Solid Edge part; units mm, degrees
sketch "Sketch1" plane through (0, 0, 0) normal (0, 0, 1) x (1, 0, 0)
  circle A0 centre (0, 0) radius 12.7
extrude "Protrusion1" add sketch "Sketch1" along normal blind 38.1
chamfer "Chamfer1" distance 1.905 angle 45 2 edges at (-12.7, 0, 0) (-12.7, 0, 38.1)
sketch "Sketch2" plane through (0, 0, 38.1) normal (0, 0, 1) x (1, 0, 0)
  line L0 (-4.1244, 7.1438) -> (4.1244, 7.1438)
  line L1 (8.2489, 0) -> (4.1244, 7.1437)
  line L2 (4.1244, -7.1437) -> (8.2489, 0)
  line L3 (-4.1244, -7.1438) -> (4.1244, -7.1438)
  line L4 (-8.2489, 0) -> (-4.1244, -7.1437)
  line L5 (-4.1244, 7.1437) -> (-8.2489, 0)
extrude "Cutout1" cut sketch "Sketch2" against normal blind 19.05
properties part number "24104263"
CAD build for the part. Positions are in the model's coordinates, mm. A direction names the side the tool comes from. Round coordinates to 2 decimals unless told otherwise and drop trailing zeros. Loops run counter-clockwise (first coordinate to the right, second up) from the corner with the lowest first, then second, coordinate; pieces in that order, holes last. Notation, with made-up numbers: M 20.25,-27 L 52.25,-27 A6 cw 52.25,-16 Z; hole C -4,63.5 d7. An arc over 180 degrees is marked long. Return JSON: item names as keys, results as strings. Group by question number.
(1) Drop flat-ended pins along their axis: P1, Ø4.5, axis at x = -4, y = -1.5, coming from the +Z side; P2, Ø1, axis at x = -8, z = 19, coming from the +Y side; P3, Ø1.5, axis at y = 7, z = 32, coming from the -X side. Give the stop position or say it passes through.
(2) Saw through at B-B, the plane x = 0. List the corners of the cut face in (y, z) (3 decimals), and give its area (3 significant figures).
(3) Tool access for faces 1 (the flat face through (0, 0, 19.05)), 2 (the conical face through (10.41, 3.28, 0.12)): list every direction of +Z, -Z, +X, -X, +Y, -Y with a clear straight run to the whole face (end or side of a thin tool).
(4) Mould opens along X. For faces 3 (the flat face through (-6.216, -3.522, 28.708)), 4 (the flat face through (7, 3, 38.1)), 5 (the cylindrical face through (-2.75, 12.4, 18.81)) say: +X half, -X half, draft (parallel to the pull), parting line (faces both ways), or undercut.
(5) Wall check: probe 1 along Z at (x, y) = (-3, -5.25); probe 2 along X at (y, z) = (-10.5, 15.5); probe 3 along X at (y, z) = (-3, 29). Give the ranges that are in metal, low to high. Write a range as [from, to].
(6) Saw through at C-C, the plane z = 13. List the corners of the cut face in (x, y).
(7) Saw through at A-A, the plane z = 23. List the corners of the cut face in (x, y), and give its area (3 significant figures).
Answer list:
{
 "1": {"P1": "z = 19.05", "P2": "y = 10.25", "P3": "x = -11.06"},
 "2": {"outline": "M -12.7,1.905 L -10.795,0 L 10.795,0 L 12.7,1.905 L 12.7,36.195 L 10.795,38.1 L 7.144,38.1 L 7.144,19.05 L -7.144,19.05 L -7.144,38.1 L -10.795,38.1 L -12.7,36.195 Z", "area": "688 mm2"},
 "3": {"face 1": "+Z", "face 2": "-Z"},
 "4": {"face 3": "undercut", "face 4": "draft", "face 5": "parting line"},
 "5": {"probe 1": "[0, 19.05]", "probe 2": "[-7.14, 7.14]", "probe 3": "[-12.34, -6.52], [6.52, 12.34]"},
 "6": {"outline": "C 0,0 d25.4"},
 "7": {"outline": "C 0,0 d25.4; hole M -8.25,0 L -4.12,-7.14 L 4.12,-7.14 L 8.25,0 L 4.12,7.14 L -4.12,7.14 Z", "area": "330 mm2"}
}
